Autodesk Inventor part; units mm, degrees
ref_plane "YZ Plane" through (0, 0, 0) normal (1, 0, 0) x (0, 1, 0)
ref_plane "XZ Plane" through (0, 0, 0) normal (0, 1, 0) x (-1, 0, 0)
ref_plane "XY Plane" through (0, 0, 0) normal (0, 0, 1) x (1, 0, 0)
sketch "Sketch1" plane through (0, 0, 0) normal (0, 0, 1) x (1, 0, 0)
  circle A0 centre (0, 0) radius 35
  dimension "d0" = 70
extrude "Extrusion1" add sketch "Sketch1" along normal blind 34
sketch "Sketch2" plane through (0, 0, 34) normal (0, 0, 1) x (1, 0, 0)
  circle A0 centre (0, 0) radius 35
  circle A1 centre (0, 0) radius 32.5
  dimension "d105" = 65
extrude "Extrusion2" cut sketch "Sketch2" against normal blind 26 contours A1
sketch "Sketch3" plane through (0, 0, 8) normal (0, 0, 1) x (1, 0, 0)
  circle A0 centre (0, 0) radius 11
  dimension "d6" = 22
extrude "Extrusion3" cut sketch "Sketch3" against normal through all
sketch "Sketch4" plane through (0, 0, 8) normal (0, 0, 1) x (1, 0, 0)
  circle A0 centre (25, 0) radius 6.5
  circle A1 centre (12.5, 21.6506) radius 6.5
  circle A2 centre (-12.5, 21.6506) radius 6.5
  circle A3 centre (-25, 0) radius 6.5
  circle A4 centre (-12.5, -21.6506) radius 6.5
  circle A5 centre (12.5, -21.6506) radius 6.5
  point P0 (0, 0)
  dimension "d9" = 13
  dimension "d10" = 25
  dimension "d13" = 360
extrude "Extrusion4" cut sketch "Sketch4" against normal blind 4
sketch "Sketch5" plane through (0, 0, 8) normal (0, 0, 1) x (1, 0, 0)
  circle A0 centre (0, 0) radius 11 construction
  circle A1 centre (25, 0) radius 2.5
  circle A2 centre (12.5, 21.6506) radius 2.5
  circle A3 centre (-12.5, 21.6506) radius 2.5
  circle A4 centre (-25, 0) radius 2.5
  circle A5 centre (-12.5, -21.6506) radius 2.5
  circle A6 centre (12.5, -21.6506) radius 2.5
  dimension "d99" = 5
  dimension "d100" = 25
  dimension "d103" = 360
extrude "Extrusion5" cut sketch "Sketch5" against normal through all
sketch "Sketch6" plane through (0, 0, 8) normal (0, 0, 1) x (1, 0, 0)
  circle A0 centre (0, 18) radius 1.5
  circle A1 centre (-15.5885, 9) radius 1.5
  circle A2 centre (-15.5885, -9) radius 1.5
  circle A3 centre (0, -18) radius 1.5
  circle A4 centre (15.5885, -9) radius 1.5
  circle A5 centre (15.5885, 9) radius 1.5
  point P0 (0, 0)
  dimension "d24" = 3
  dimension "d25" = 18
  dimension "d28" = 360
extrude "Extrusion6" cut sketch "Sketch6" against normal through all
sketch "Sketch27" plane through (0, 0, 8) normal (0, 0, 1) x (1, 0, 0)
  circle A0 centre (-15.5885, -9) radius 1.5 construction
  circle A1 centre (-15.5885, -9) radius 13.5 construction
  circle A2 centre (15.5885, -9) radius 1.5 construction
  circle A3 centre (15.5885, -9) radius 13.5 construction
  circle A4 centre (0, -18) radius 1.5
  circle A5 centre (-12.5, -21.6506) radius 6.5 construction
  circle A6 centre (0, 0) radius 11 construction
  arc A7 (-6.5519, -19.0295) -> (-2.2059, -10.7766) centre (-15.5885, -9) ccw
  arc A8 (2.2059, -10.7766) -> (6.5519, -19.0295) centre (15.5885, -9) ccw
  circle A9 centre (12.5, -21.6506) radius 6.5 construction
  circle A10 centre (0, -18) radius 13.5 construction
  arc A11 (6.5519, -19.0295) -> (9.6157, -27.4757) centre (12.5, -21.6506) ccw
  arc A12 (-9.6157, -27.4757) -> (-6.5519, -19.0295) centre (-12.5, -21.6506) ccw
  arc A13 (-9.6157, -27.4757) -> (9.6157, -27.4757) centre (0, -18) ccw
  arc A14 (-2.2059, -10.7766) -> (2.2059, -10.7766) centre (0, 0) ccw
  dimension "d106" = 27
  dimension "d107" = 27
  dimension "d108" = 27
extrude "Extrusion24" add sketch "Sketch27" along normal blind 5
properties part number "Base" material "ABS Plastic"
For this review, take the finished solid that the model builds, in its own axes (mm). A direction names the side the tool comes from. Give positions to 0.01 mm unless a question says otherwise; leave off trailing zeros. Write each loop counter-clockwise with the first axis right and the second up, starting at its lowest first coordinate (ties: lowest second). Pieces come first, ordered by that corner, then holes. Notation, with made-up numbers: M 14,55 L 44,55 A20 ccw 44,86 Z; hole C -36,-33 d11. An arc over 180 degrees is marked long. One line per item, written item: value.
1) For P1, Ø1, axis at x = -16, z = 29, coming from the +Y side; P2, Ø10.5, axis at x = 11, y = 23.5, coming from the +Z side; P3, Ø21, axis at x = 4, y = -21, coming from the +Z side, all flat-tipped, find the tip position at first contact; note any pin that passes through.
Results are:
P1: stops at y = 31.38
P2: stops at z = 8
P3: stops at z = 13
2) Take a section at A-A, the plane z = 12. Write out the cut boundary in (x, y).
Results are:
outline: C 0,0 d70; M -9.62,-27.48 A13.5 ccw 9.62,-27.48 A6.5 cw 6.55,-19.03 A13.5 cw 2.21,-10.78 A11 cw -2.21,-10.78 A13.5 cw -6.55,-19.03 A6.5 cw Z; hole C 0,0 d65; hole C 0,-18 d3
3) The part is to be moulded in two halves that separate along Y. For faces 3 (the cylindrical face through (-14.896, 7.669, 4.056)), 4 (the flat face through (-8, 8, 0)), say which applies: +Y half, -Y half, draft (parallel to the pull), parting line (faces both ways), or undercut.
Results are:
face 3: undercut
face 4: draft
4) Take a section at C-C, the plane y = 18. Write out the cut boundary in (x, z), then the cut area to 3 significant figures.
Results are:
outline: M -30.02,0 L -1.5,0 L -1.5,8 L -7.12,8 L -7.12,4 L -17.88,4 L -17.88,8 L -27.06,8 L -27.06,34 L -30.02,34 Z; M 1.5,0 L 30.02,0 L 30.02,34 L 27.06,34 L 27.06,8 L 17.88,8 L 17.88,4 L 7.12,4 L 7.12,8 L 1.5,8 Z
area: 524 mm²
5) Take a section at D-D, the plane x = 12.5. Write out the cut boundary in (y, z), then the cut area to 3 significant figures.
Results are:
outline: M -32.69,0 L -24.15,0 L -24.15,4 L -28.15,4 L -28.15,8 L -30,8 L -30,34 L -32.69,34 Z; M -19.15,0 L 19.15,0 L 19.15,4 L 15.15,4 L 15.15,8 L -15.15,8 L -15.15,4 L -19.15,4 Z; M 24.15,0 L 32.69,0 L 32.69,34 L 30,34 L 30,8 L 28.15,8 L 28.15,4 L 24.15,4 Z
area: 519 mm²
6) Take a section at B-B, the plane x = -25. Write out the cut boundary in (y, z), then the cut area to 3 significant figures.
Results are:
outline: M -24.49,0 L -2.5,0 L -2.5,4 L -6.5,4 L -6.5,8 L -20.77,8 L -20.77,34 L -24.49,34 Z; M 2.5,0 L 24.49,0 L 24.49,34 L 20.77,34 L 20.77,8 L 6.5,8 L 6.5,4 L 2.5,4 Z
area: 514 mm²
7) For faces 1 (the flat face through (0, -23, 13)), 2 (the cylindrical face through (12, -24.1, 2)), list the 3-axis set-ups (+Z, -Z, +X, -X, +Y, -Y) from which the entire face can be reached by the end or side of a thin tool; tool diameter is ignored.
Results are:
face 1: +Z
face 2: +Z, -Z
8) For line 1 (Y direction, x = 0, z = 7); line 2 (X direction, y = 21.5, z = 7); line 3 (Z direction, x = 31, y = 7.5), list the stretches that pass through material, from the lowest coordinate up. Write a range as from..to.
Results are:
line 1: y = -35..-19.5, -16.5..-11, 11..16.5, 19.5..35
line 2: x = -27.62..-19, -6..6, 19..27.62
line 3: z = 0..8
